Autodesk Inventor part; units mm, degrees
ref_plane "YZ Plane" through (0, 0, 0) normal (1, 0, 0) x (0, 1, 0)
ref_plane "XZ Plane" through (0, 0, 0) normal (0, 1, 0) x (-1, 0, 0)
ref_plane "XY Plane" through (0, 0, 0) normal (0, 0, 1) x (1, 0, 0)
sketch "Sketch1" plane through (0, 0, 0) normal (0, 1, 0) x (-1, 0, 0)
  line L0 (-3.6662, 6.35) -> (3.6662, 6.35)
  line L1 (3.6662, 6.35) -> (7.3323, 0)
  line L2 (7.3323, 0) -> (3.6662, -6.35)
  line L3 (3.6662, -6.35) -> (-3.6662, -6.35)
  line L4 (-3.6662, -6.35) -> (-7.3323, 0)
  line L5 (-7.3323, 0) -> (-3.6662, 6.35)
  circle A0 centre (0, 0) radius 2.54
  dimension "d0" = 12.7
  dimension "d1" = 5.08
extrude "Extrusion1" add sketch "Sketch1" along normal blind 76.2
sketch "Sketch2" plane through (0, 76.2, 0) normal (0, 1, 0) x (1, 0, 0)
  line L0 (-3.6662, 6.35) -> (3.6662, 6.35)
  arc A0 (-1.5875, 6.35) -> (1.5875, 6.35) centre (0, 6.35) ccw
  line L1 (-1.5875, 6.35) -> (1.5875, 6.35)
  dimension "d4" = 1.5875
extrude "Extrusion2" cut sketch "Sketch2" against normal through all
pattern_circular "Circular Pattern1" count 6 over 360 about axis through (0, 0, 0) along (0, 1, 0) of "Extrusion2"
properties part number "BatteryStandoff" material "Aluminum-6061"
Can you work these out from the model? Positions are in its coordinate system, mm. Coordinates: 2 decimals unless noted, no trailing zeros. Loops run counter-clockwise (first coordinate to the right, second up) from the corner with the lowest first, then second, coordinate; pieces in that order, holes last.
Item 1: Suppose I cut it at B-B (x = 0). Please give me the cut outline in (y, z), then the cut area to 3 significant figures.
Answers below:
outline: (0, -4.76) - (76.2, -4.76) - (76.2, -2.54) - (0, -2.54) - close; (0, 2.54) - (76.2, 2.54) - (76.2, 4.76) - (0, 4.76) - close
area: 339 mm2
Item 2: Please list where these lines run through material, in increasing order: L1, parallel to Z at x = 0, y = 53.5; L2, parallel to Z at x = 0.75, y = 37; L3, parallel to X at y = 29, z = 1.
Answers below:
L1: z = -4.76 to -2.54, 2.54 to 4.76
L2: z = -4.95 to -2.43, 2.43 to 4.95
L3: x = -6.75 to -2.33, 2.33 to 6.75
Item 3: I'm going to push flat-ended pins straight in: pin 1 (5 mm diameter, centred on y = 30.5, z = -3.5, fed in from -X); pin 2 (2 mm diameter, centred on x = -5.5, y = 23.5, fed in from -Z). Where does each tip first touch, or does it pass through?
Answers below:
pin 1: stops at x = -6.75
pin 2: stops at z = -4.91
Item 4: Suppose I cut it at C-C (z = 0.75). Please give me the cut outline in (x, y), then the cut area to 3 significant figures.
Answers below:
outline: (-6.9, 0) - (-2.43, 0) - (-2.43, 76.2) - (-6.9, 76.2) - close; (2.43, 0) - (6.9, 0) - (6.9, 76.2) - (2.43, 76.2) - close
area: 682 mm2
Item 5: If we mould it in two halves opening along X, with no side actions, what happens to faces 1 (the face through (6.805, 37.567, -0.913)), 2 (the face through (4.142, 38.633, 2.351)), 3 (the face through (-6.82, 37.57, -0.89))? For each: released by +X, released by -X, zero draft, split by the parting line, or undercut.
Answers below:
face 1: released by +X
face 2: undercut
face 3: released by -X
